Read the model definition and answer for the solid it produces. Units are mm, in the model's axes. A direction names the side the tool comes from. Round coordinates to 2 decimals unless told otherwise and drop trailing zeros. Loops run counter-clockwise (first coordinate to the right, second up) from the corner with the lowest first, then second, coordinate; pieces in that order, holes last. Notation, with made-up numbers: (-26.5, 7.25) -> (21.5, 7.25) arc R25 ccw to (21.5, 34.25) -> close; hole circle Ø7 at (-24, 52.5). An arc over 180 degrees is marked (long way). Put each result on its own line as item: value.
from build123d import *

# Parameters (mm, degrees)
F0_R     = 17.25
F0_R_2   = 5.9
F1_DEPTH = 32.5
F3_DEPTH = 0.5
F4_SIZE  = 1


with BuildPart() as f1:
    # F0 (on Front) → F1 (new body)
    with BuildSketch(Plane.XZ):
        Circle(F0_R)
        Circle(F0_R_2, mode=Mode.SUBTRACT)
    extrude(amount=F1_DEPTH)

    # F2 (on face) → F3 (cut)
    with BuildSketch(Plane.XZ.offset(32.5)):
        with BuildLine():
            ThreePointArc((-5.9, 0), (0, 5.9), (5.9, 0))
            Line((5.9, 0), (17.25, 0))
            ThreePointArc((17.25, 0), (0, 17.25), (-17.25, 0))
            Line((-17.25, 0), (-5.9, 0))
        make_face()
    extrude(amount=-F3_DEPTH, mode=Mode.SUBTRACT)

    # F4
    f4_edges = [f1.edges().sort_by_distance(p)[0] for p in [
        (-5.9, 0, 0),
    ]]
    chamfer(f4_edges, length=F4_SIZE)


solid = f1.part
Item 1: Flat-ended cylindrical pins translate along their axes: pin 1 Ø3 at (x, y) = (8.5, -15.5) entering from +Z; pin 2 Ø3 at (x, y) = (-8, -11) entering from -Z; pin 3 Ø5 at (x, z) = (7.5, 8) entering from -Y. Find the tip coordinate at first contact, or state that the pin passes through.
Derived:
pin 1: stops at z = 15.77
pin 2: stops at z = -15.98
pin 3: stops at y = -32
Item 2: Which of the six approach directions +Z, -Z, +X, -X, +Y, -Y give full straight-line access (tool end or side, diameter ignored) to faces 1 (the flat face through (0, -32, 9)), 2 (the flat face through (0, -32.5, -9))?
Derived:
face 1: +Z, +X, -X, -Y
face 2: +Z, -Z, +X, -X, -Y
Item 3: Find the intervals of material crossed by line 1 along Z through (x, y) = (0, -24); line 2 along X through (y, z) = (-22.5, -4.5); line 3 along Y through (x, z) = (-5.5, 4.5), in increasing order.
Derived:
line 1: z = -17.25 to -5.9, 5.9 to 17.25
line 2: x = -16.65 to -3.82, 3.82 to 16.65
line 3: y = -32 to 0
Item 4: The part is cut by section C-C (x = -14). Determine the outline of the cut face in (y, z), then the cut area to 3 significant figures.
Derived:
outline: (-32.5, -10.08) -> (0, -10.08) -> (0, 10.08) -> (-32, 10.08) -> (-32, 0) -> (-32.5, 0) -> close
area: 650 mm^2
Item 5: The part is cut by section A-A (x = 0). Determine the outline of the cut face in (y, z).
Derived:
outline: (-32.5, -17.25) -> (0, -17.25) -> (0, -6.9) -> (-1, -5.9) -> (-32.5, -5.9) -> close; (-32, 5.9) -> (-1, 5.9) -> (0, 6.9) -> (0, 17.25) -> (-32, 17.25) -> close
Item 6: The part is cut by section D-D (z = 9). Determine the outline of the cut face in (x, y).
Derived:
outline: (-14.72, -32) -> (14.72, -32) -> (14.72, 0) -> (-14.72, 0) -> close
Item 7: The part is cut by section B-B (y = -10). Determine the outline of the cut face in (x, z).
Derived:
outline: circle Ø34.5 at (0, 0); hole circle Ø11.8 at (0, 0)
Item 8: For a pull along X with two mould halves and no side action, classify faces 3 (the cylindrical face through (16.453, -16.022, 5.181)), 4 (the cylindrical face through (-5.894, -16.53, 0.259)), 5 (the flat face through (-0.2, 0, -7.4)) as pulls with the +X half, pulls with the -X half, needs draft (parallel to the pull), parting line crosses it, or undercut.
Derived:
face 3: parting line crosses it
face 4: undercut
face 5: needs draft
